Input: dimensioned drawing with shaded views. Units: mm. Origin: part minimum x, y, z. Coordinates: 2 decimals unless noted, no trailing zeros. Write each loop counter-clockwise with the first axis right and the second up, starting at its lowest first coordinate (ties: lowest second). Pieces come first, ordered by that corner, then holes. Notation, with made-up numbers: (-21, -29) - (6, -29) arc R25 cw to (6, -12) - close; hole circle Ø10 at (-18, 42). An arc over 180 degrees is marked (long way). One line per question, with ' | ' between items.
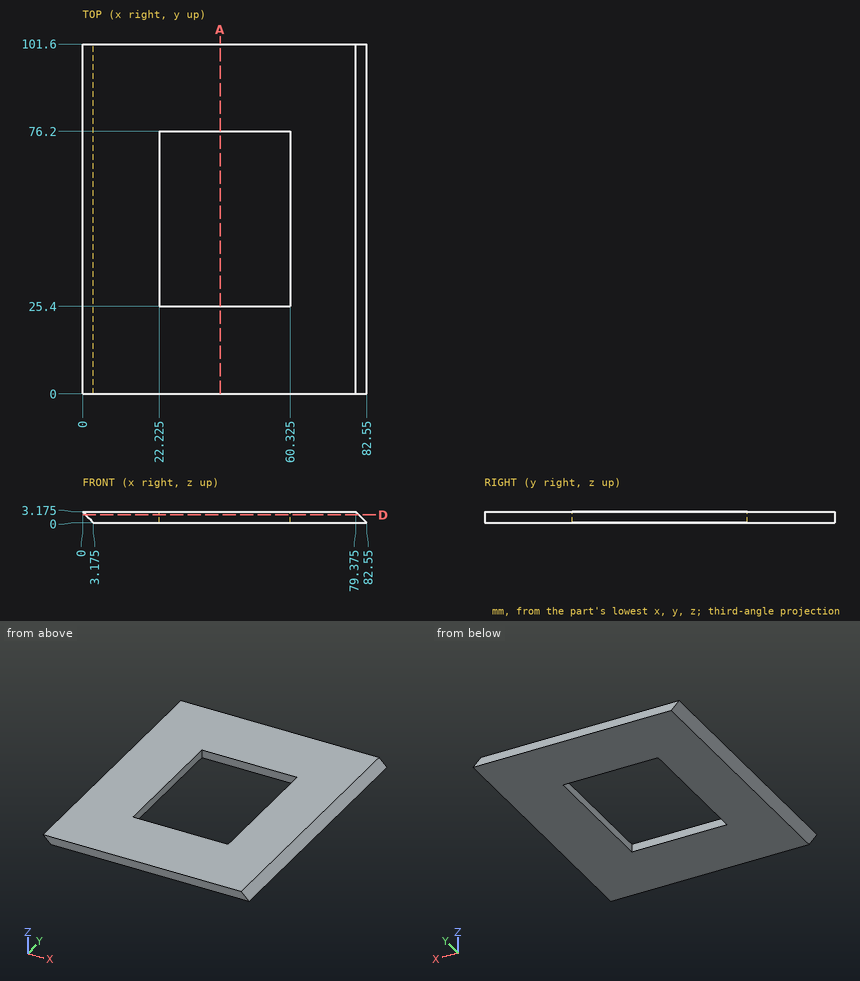
Item 1: Cut plane A-A on x = 40. Return loops of the section in (y, z) (3 decimals), and give its area (3 significant figures).
Check sheet entries:
outline: (0, 0) - (25.4, 0) - (25.4, 3.175) - (0, 3.175) - close; (76.2, 0) - (101.6, 0) - (101.6, 3.175) - (76.2, 3.175) - close | area: 161 mm²
Item 2: Ray query, line 1 along Y through (x, z) = (41.5, 0.9); line 2 along X through (y, z) = (30, 0.25) (3 decimals); line 3 along X through (y, z) = (69, 2.5) (3 decimals). Return the intervals inside material, ascending. Write a range as [from, to].
Check sheet entries:
line 1: [0, 25.4], [76.2, 101.6] | line 2: [2.925, 22.225], [60.325, 82.3] | line 3: [0.675, 22.225], [60.325, 80.05]
Item 3: Cut plane D-D on z = 2.25. Return loops of the section in (x, y) (3 decimals), and give its area (3 significant figures).
Check sheet entries:
outline: (0.925, 0) - (80.3, 0) - (80.3, 101.6) - (0.925, 101.6) - close; hole (22.225, 25.4) - (60.325, 25.4) - (60.325, 76.2) - (22.225, 76.2) - close | area: 6,130 mm²
Item 4: Pin query (flat end, axial travel): pin 1 Ø1.6 at (y, z) = (62, 1.5) entering from +X. Return the tip coordinate at first contact, or that it passes through.
Check sheet entries:
pin 1: x = 81.85
